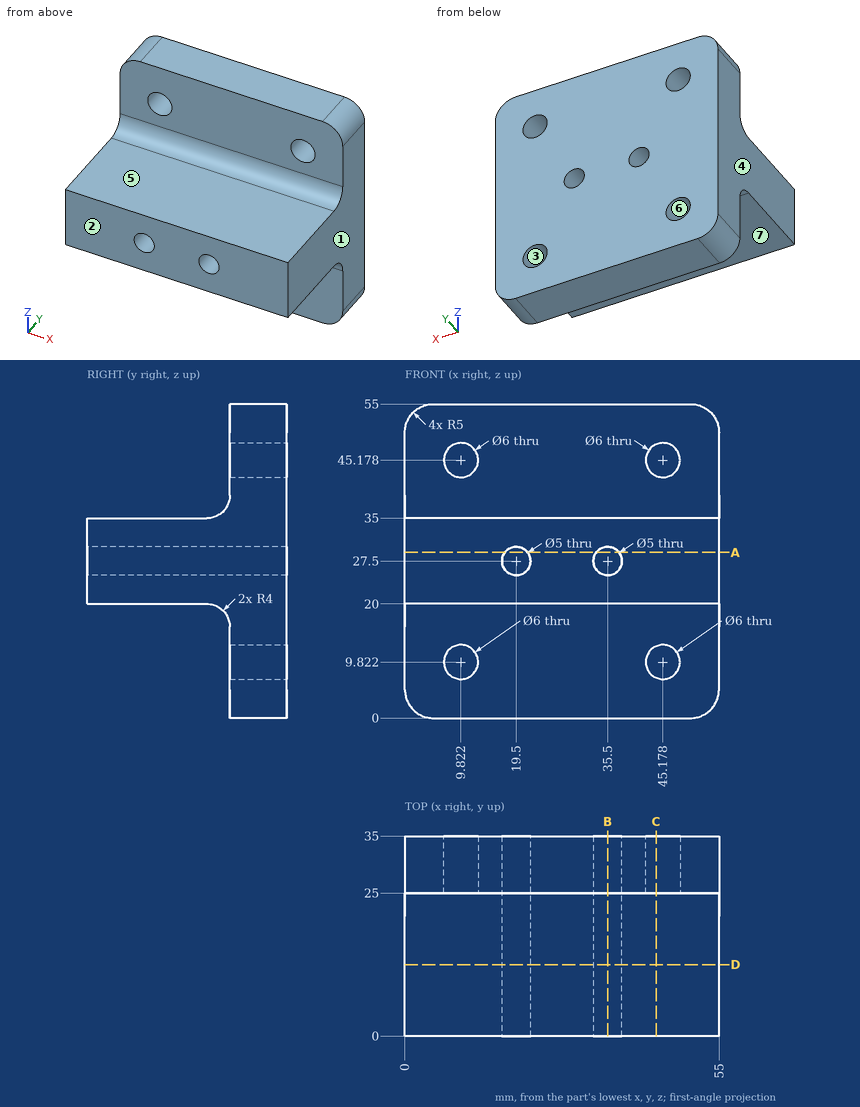
Study the drawing (mm; zero at the part's minimum x, y, z) and answer. A direction names the side the tool comes from. Coordinates: 2 decimals unless noted, no trailing zeros. Write each loop counter-clockwise with the first axis right and the second up, starting at its lowest first coordinate (ties: lowest second). Pieces come first, ordered by that corner, then holes. Notation, with made-up numbers: (72.25, -8) - (116.25, -8) arc R37 cw to (116.25, 30) - close; hole circle Ø5 at (-19.5, -30.75). An arc over 180 degrees is marked (long way). Return JSON: item names as keys, results as strings. Group by question number.
1. Given pin 1 (5.5 mm diameter, centred on x = 9.82, z = 9.82, fed in from -Y); pin 2 (8 mm diameter, centred on x = 35.5, z = 47, fed in from -Y); pin 3 (10.5 mm diameter, centred on x = 26, y = 12, fed in from +Z), each flat-ended and moving along its own axis, determine where each tip first touches the part or whether it passes through.
2. A cutting plane is placed at C-C, the plane x = 44. Determine the outline of the cut face in (y, z).
3. Determine the mould class of the marked faces 1, 2, 3 and 4 for opening direction X: released by +X, released by -X, zero draft, split by the parting line, or undercut.
4. A cutting plane is placed at D-D, the plane y = 12.5. Determine the outline of the cut face in (x, z), plus the area to 3 significant figures.
5. Straight lines are drawn through the part: L1, parallel to X at y = 15, z = 27.5; L2, parallel to Y at x = 41, z = 51; L3, parallel to Z at x = 25.5, y = 17. For each, find the intervals that lie inside material, in ascending order.
6. Which of the six approach directions +Z, -Z, +X, -X, +Y, -Y give full straight-line access (tool end or side, diameter ignored) to the marked faces 5, 6 and 7?
7. A cutting plane is placed at B-B, the plane x = 35.5. Determine the outline of the cut face in (y, z).
8. A cutting plane is placed at A-A, the plane z = 29. Determine the outline of the cut face in (x, y), plus the area to 4 significant figures.
Ans:
{
 "1": {"pin 1": "through", "pin 2": "y = 25", "pin 3": "z = 35"},
 "2": {"outline": "(0, 20) - (21, 20) arc R4 cw to (25, 16) - (25, 12.58) - (35, 12.58) - (35, 42.42) - (25, 42.42) - (25, 39) arc R4 cw to (21, 35) - (0, 35) - close; (25, 0) - (35, 0) - (35, 7.06) - (25, 7.06) - close; (25, 47.94) - (35, 47.94) - (35, 55) - (25, 55) - close"},
 "3": {"face 1": "released by +X", "face 2": "zero draft", "face 3": "undercut", "face 4": "released by -X"},
 "4": {"outline": "(0, 20) - (55, 20) - (55, 35) - (0, 35) - close; hole circle Ø5 at (19.5, 27.5); hole circle Ø5 at (35.5, 27.5)", "area": "786 mm²"},
 "5": {"L1": "0 to 17, 22 to 33, 38 to 55", "L2": "25 to 35", "L3": "20 to 35"},
 "6": {"face 5": "+Z, +X, -X, -Y", "face 6": "+Y, -Y", "face 7": "-Z, +X, -X, -Y"},
 "7": {"outline": "(0, 20) - (21, 20) arc R4 cw to (25, 16) - (25, 0) - (35, 0) - (35, 25) - (0, 25) - close; (0, 30) - (35, 30) - (35, 55) - (25, 55) - (25, 39) arc R4 cw to (21, 35) - (0, 35) - close"},
 "8": {"outline": "(0, 0) - (17.5, 0) - (17.5, 35) - (0, 35) - close; (21.5, 0) - (33.5, 0) - (33.5, 35) - (21.5, 35) - close; (37.5, 0) - (55, 0) - (55, 35) - (37.5, 35) - close", "area": "1,645 mm²"}
}
